The listing builds one solid part. Answer for the finished solid, in the listing's coordinates (mm). A direction names the side the tool comes from. Round coordinates to 2 decimals unless told otherwise and drop trailing zeros. Loops run counter-clockwise (first coordinate to the right, second up) from the corner with the lowest first, then second, coordinate; pieces in that order, holes last. Notation, with made-up numbers: (41, 9.25) - (45, 9.25) arc R7 cw to (45, 21.25) - close; hole circle Ø9 at (61, 77.5). An arc over 180 degrees is marked (long way). Write item = value, one per line. Start each with the question number.
1) For a pull along Y with two mould halves and no side action, classify faces 4 (the flat face through (-20, 54, 42)), 5 (the flat face through (-20, 27, 85)), 6 (the cylindrical face through (-22.54, 36.61, 76.39)) as released by +Y, released by -Y, zero draft, split by the parting line, or undercut.
2) Given pin 1 Ø1.8 at (y, z) = (36, 44.5) entering from -X; pin 2 Ø1 at (x, z) = (-23.5, 57.5) entering from -Y; pin 3 Ø5 at (y, z) = (11, 60) entering from +X, each flat-ended and moving along its own axis, determine where each tip first touches the part or whether it passes through.
3) Section A-A, the plane z = 60 is taken. Determine the outline of the cut face in (x, y), and give its area (3 significant figures).
4) Section B-B, the plane y = 18 is taken. Determine the outline of the cut face in (x, z).
5) Section D-D, the plane x = -13.5 is taken. Determine the outline of the cut face in (y, z), and give its area (3 significant figures).
6) Section C-C, the plane x = -23.5 is taken. Determine the outline of the cut face in (y, z).
7) Straight lines are drawn through the part: line 1 along Z through (x, y) = (-23.6, 35); line 2 along Y through (x, z) = (-15.75, 53.5); line 3 along Z through (x, y) = (-16.25, 34). For each, find the intervals that lie inside material, in ascending order.
8) A tool of negligible diameter and unlimited length cuts with its end or side. For faces 1 (the flat face through (-13, 27, 38)), 2 (the cylindrical face through (-17.465, 25.568, 70.906)), 3 (the flat face through (-20, 28.3, 73.7)), from which of +Z, -Z, +X, -X, +Y, -Y can it reach the whole face along a straight path? Write none if from no direction.
from build123d import *

# Parameters (mm, degrees)
PAD_DEPTH             = 38
SKETCH_W              = 10
SKETCH_H              = 54
PAD001_DEPTH          = 85
SKETCH002_R           = 10
POCKET_DEPTH          = 25.001
SKETCH003_R           = 1.5
POCKET001_DEPTH       = 218.62811
POLARPATTERN_COUNT    = 3
SKETCH004_R           = 3
POCKET002_DEPTH       = 5
POLARPATTERN001_COUNT = 3
SKETCH005_R           = 11
POCKET003_DEPTH       = 20


with BuildPart() as part:
    # Sketch001 → Pad (new body)
    with BuildSketch(Plane.XY):
        Polygon((-15, 0), (-15, 14.5), (-10, 12), (-10, 42), (-15, 39.5), (-15, 54), (-25, 54), (-25, 0), align=None)
    extrude(amount=PAD_DEPTH)

    # Sketch → Pad001 (join)
    with BuildSketch(Plane.XY):
        with Locations((-20, 27)):
            Rectangle(SKETCH_W, SKETCH_H)
    extrude(amount=PAD001_DEPTH)

    # Sketch002 → Pocket (cut, through all)
    with BuildSketch(Plane.YZ):
        with Locations((27, 60)):
            Circle(SKETCH002_R)
    extrude(amount=-POCKET_DEPTH, mode=Mode.SUBTRACT)

    # Sketch003 → Pocket001 (cut, through all)
    with BuildSketch(Plane(origin=(-25, 27, 60), x_dir=(0, 1, 0), z_dir=(1, 0, 0))):
        with Locations((0, 15)):
            Circle(SKETCH003_R)
        with Locations((-16, 0)):
            Circle(SKETCH003_R)
    pocket001 = extrude(amount=POCKET001_DEPTH, mode=Mode.SUBTRACT)

    # PolarPattern: Pocket001 ×3 about axis
    polarpattern_axis = Axis((-25, 27, 60), (1, 0, 0))
    for i in range(1, POLARPATTERN_COUNT):
        add(pocket001.rotate(polarpattern_axis, i * 360 / POLARPATTERN_COUNT), mode=Mode.SUBTRACT)

    # Sketch004 → Pocket002 (cut)
    with BuildSketch(Plane(origin=(-25, 27, 60), x_dir=(0, 1, 0), z_dir=(1, 0, 0))):
        with Locations((0, 15)):
            Circle(SKETCH004_R)
        with Locations((-16, 0)):
            Circle(SKETCH004_R)
    pocket002 = extrude(amount=POCKET002_DEPTH, mode=Mode.SUBTRACT)

    # PolarPattern001: Pocket002 ×3 about axis
    polarpattern001_axis = Axis((-25, 27, 60), (1, 0, 0))
    for i in range(1, POLARPATTERN001_COUNT):
        add(pocket002.rotate(polarpattern001_axis, i * 360 / POLARPATTERN001_COUNT), mode=Mode.SUBTRACT)

    # Sketch005 → Pocket003 (cut)
    with BuildSketch(Plane.YZ):
        with Locations((27, 60)):
            Circle(SKETCH005_R)
    extrude(amount=-POCKET003_DEPTH, mode=Mode.SUBTRACT)


solid = part.part
Geometry check:
q1.face_4 = released by +Y
q1.face_5 = zero draft
q1.face_6 = undercut
q2.pin_1 = -20
q2.pin_2 = 0
q2.pin_3 = -15
q3.outline = (-25, 0) - (-15, 0) - (-15, 9.5) - (-20, 9.5) - (-20, 8) - (-25, 8) - close; (-25, 14) - (-20, 14) - (-20, 12.5) - (-15, 12.5) - (-15, 16) - (-20, 16) - (-20, 17) - (-25, 17) - close; (-25, 37) - (-20, 37) - (-20, 38) - (-15, 38) - (-15, 54) - (-25, 54) - close
q3.area = 285 mm2
q4.outline = (-25, 0) - (-10, 0) - (-10, 38) - (-15, 38) - (-15, 53.68) - (-20, 53.68) - (-20, 55.64) - (-25, 55.64) - close; (-25, 64.36) - (-20, 64.36) - (-20, 66.32) - (-15, 66.32) - (-15, 85) - (-25, 85) - close
q5.outline = (13.75, 0) - (40.25, 0) - (40.25, 38) - (13.75, 38) - close
q5.area = 1,010 mm2
q6.outline = (0, 0) - (54, 0) - (54, 85) - (0, 85) - close; hole circle Ø6 at (11, 60); hole circle Ø6 at (14.01, 52.5); hole circle Ø20 at (27, 60); hole circle Ø6 at (27, 75); hole circle Ø6 at (35, 46.14); hole circle Ø6 at (35, 73.86); hole circle Ø6 at (39.99, 52.5)
q7.line_1 = 0 to 43.14, 49.14 to 54, 66 to 70.86, 76.86 to 85
q7.line_2 = 0 to 12.89, 15.13 to 18.13, 35.87 to 38.87, 41.11 to 54
q7.line_3 = 0 to 45.03, 47.26 to 51.51, 68.49 to 72.74, 74.97 to 85
q8.face_1 = +Z, +X, +Y, -Y
q8.face_2 = +X
q8.face_3 = -X
